Can you work these out from the drawing? Everything is in mm from the part's minimum corner. A direction names the side the tool comes from. Round coordinates to 2 decimals unless told otherwise and drop trailing zeros. Order: outer loops, then holes, each group sorted by start corner. A loop starts at its lowest first (then second) coordinate and runs counter-clockwise, first axis right, second up. Notation, with made-up numbers: (2.5, 45.25) -> (18.5, 45.25) arc R22 cw to (18.5, 57.25) -> close; hole circle Ø6 at (44, 47). An arc over 180 degrees is marked (long way). One line per item, written item: value.
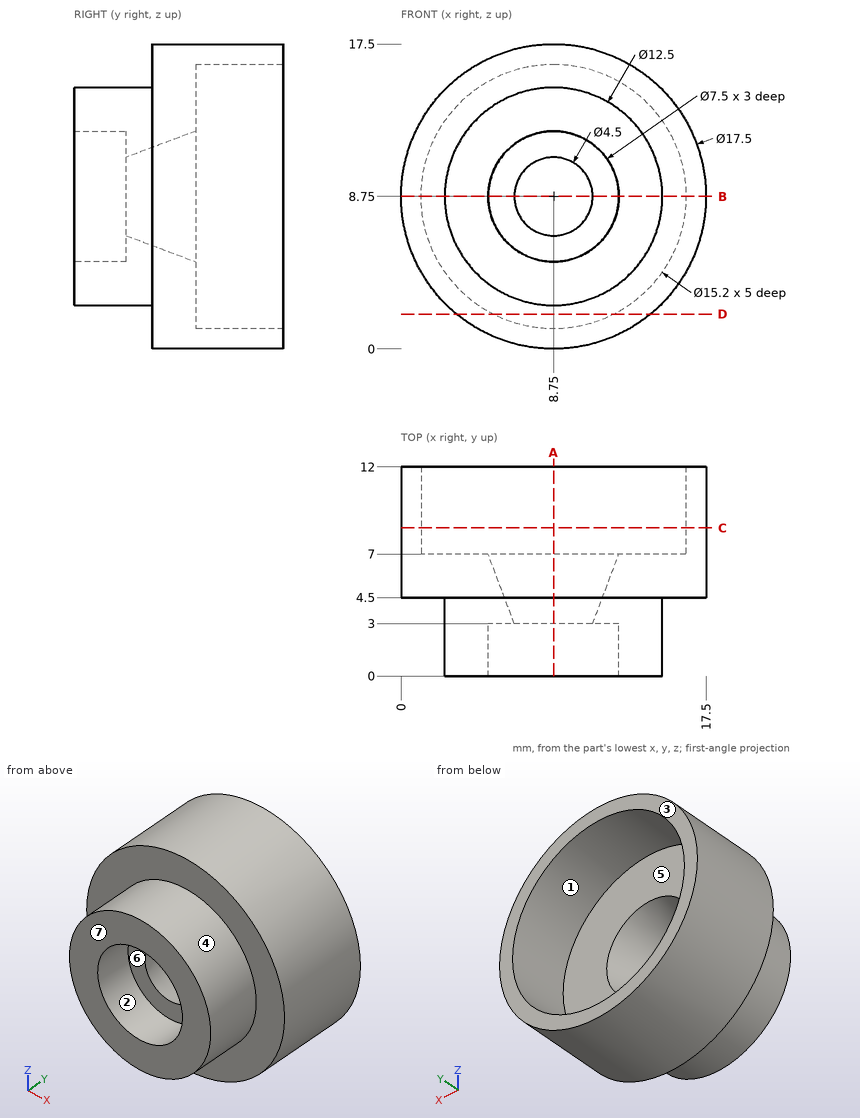
Q1. I want a section at A-A on x = 8.75. List the corners of the cut face in (y, z) for me, plus the area to 3 significant figures.
Answers below:
outline: (0, 2.5) -> (4.5, 2.5) -> (4.5, 0) -> (12, 0) -> (12, 1.15) -> (7, 1.15) -> (7, 5) -> (3, 6.5) -> (3, 5) -> (0, 5) -> close; (0, 12.5) -> (3, 12.5) -> (3, 11) -> (7, 12.5) -> (7, 16.35) -> (12, 16.35) -> (12, 17.5) -> (4.5, 17.5) -> (4.5, 15) -> (0, 15) -> close
area: 65.0 mm^2
Q2. Please list where these lines run through material, in increasing order: line 1 along X through (y, z) = (2.4, 8.75); line 2 along X through (y, z) = (8.75, 8.75); line 3 along Y through (x, z) = (13.5, 6.25).
Answers below:
line 1: 2.5 to 5, 12.5 to 15
line 2: 0 to 1.15, 16.35 to 17.5
line 3: 0 to 7
Q3. I want a section at B-B on z = 8.75. List the corners of the cut face in (x, y) for me.
Answers below:
outline: (0, 4.5) -> (2.5, 4.5) -> (2.5, 0) -> (5, 0) -> (5, 3) -> (6.5, 3) -> (5, 7) -> (1.15, 7) -> (1.15, 12) -> (0, 12) -> close; (11, 3) -> (12.5, 3) -> (12.5, 0) -> (15, 0) -> (15, 4.5) -> (17.5, 4.5) -> (17.5, 12) -> (16.35, 12) -> (16.35, 7) -> (12.5, 7) -> close
Q4. I want a section at D-D on z = 2. List the corners of the cut face in (x, y) for me.
Answers below:
outline: (3.18, 4.5) -> (14.32, 4.5) -> (14.32, 12) -> (12.24, 12) -> (12.24, 7) -> (5.26, 7) -> (5.26, 12) -> (3.18, 12) -> close
Q5. On a 3-axis mill with a long thin cutter (end or side, diameter ignored), from which of +Z, -Z, +X, -X, +Y, -Y can I reach the whole of each face in a straight line? I mean the marked faces 1, 2 and 3. Say none if no direction works.
Answers below:
face 1: +Y
face 2: -Y
face 3: +Z, -Z, +X, -X, +Y
Q6. We'd pull the mould along X, two halves only. Please class the marked faces 4, 5, 6 and 7: released by +X, released by -X, zero draft, split by the parting line, or undercut.
Answers below:
face 4: split by the parting line
face 5: undercut
face 6: undercut
face 7: zero draft
Q7. I want a section at C-C on y = 8.5. List the corners of the cut face in (x, z) for me.
Answers below:
outline: circle Ø17.5 at (8.75, 8.75); hole circle Ø15.2 at (8.75, 8.75)
Q8. Will these pins go through, and if not, where does the flat tip stop? pin 1 Ø1.5 at (x, y) = (5.5, 6) entering from -Z; pin 2 Ø4 at (y, z) = (10.5, 15.5) entering from -X; pin 3 Ø1 at (x, y) = (6, 4.5) entering from -Z.
Answers below:
pin 1: z = 0.36
pin 2: x = 1.4
pin 3: z = 0.29
